Design review of the part built by this model. Coordinates are the model's own, in mm. Round coordinates to 2 decimals unless told otherwise and drop trailing zeros. Write each loop counter-clockwise with the first axis right and the second up, starting at its lowest first coordinate (ties: lowest second). Pieces come first, ordered by that corner, then holes. Notation, with made-up numbers: (55.25, 67.5) -> (61.25, 67.5) arc R23 cw to (61.25, 83.5) -> close; hole circle Ø9 at (-37, 53.5). An arc over 180 degrees is marked (long way). One line per question, with ' | ' between items. Start each with the question number.
1) Consider section A-A (y = -7). Give the boundary of the cut face in (x, z), then the cut area to 3 significant figures.
2) Consider section D-D (y = -53). Give the boundary of the cut face in (x, z).
3) Consider section C-C (x = -2.5). Give the boundary of the cut face in (y, z), then the cut area to 3 significant figures.
4) Mouldability with a two-part tool opening along X and no side actions: class faces 1 (the flat face through (-2, -35, 6)), 2 (the cylindrical face through (-51.225, -1.504, 3.052)), 3 (the flat face through (43.21, -29.65, -40.92)) as +X half, -X half, draft (parallel to the pull), parting line (faces both ways), or undercut.
5) Consider section B-B (z = 1). Give the boundary of the cut face in (x, y).
6) Insertion check: pin 1 Ø25 at (x, z) = (-9, 15.5) entering from -Y; pin 2 Ø4 at (x, y) = (-33.5, -37.5) entering from -Z. Each pin has a flat end and moves straight along its axis. Give the tip position at first contact, or say it passes through.
7) For probe 1 along Y at (x, z) = (-12.5, -2); probe 2 along Z at (x, y) = (17, -49); probe 3 along X at (y, z) = (-54, 8.5), list the stretches that pass through material, from the lowest coordinate up.
```python
from build123d import *

# Parameters (mm, degrees)
F1_DEPTH = 60
F2_R     = 5
F3_R     = 25
F4_DEPTH = 25


with BuildPart() as f1:
    # F0 (on Front) → F1 (new body)
    with BuildSketch(Plane.XZ):
        with BuildLine():
            Line((33.469399, 53.402335), (-27.650935, 53.402335))
            ThreePointArc((-27.650935, 53.402335), (-45.328605, 46.080005), (-52.650935, 28.402335))
            Line((-52.650935, 28.402335), (-52.650935, -21.597665))
            ThreePointArc((-52.650935, -21.597665), (-45.328605, -39.275334), (-27.650935, -46.597665))
            Line((-27.650935, -46.597665), (39.180679, -46.597665))
            Line((39.180679, -46.597665), (47.349065, -35.087663))
            Line((47.349065, -35.087663), (47.349065, 40.44798))
            Line((47.349065, 40.44798), (33.469399, 53.402335))
        make_face()
    extrude(amount=F1_DEPTH)

    # F2
    f2_edges = [f1.edges().sort_by_distance(p)[0] for p in [
        (40.409232, -60, 46.925158),
        (2.909232, -60, 53.402335),
        (-45.328605, -60, 46.080005),
        (-52.650935, -60, 3.402335),
        (-45.328605, -60, -39.275334),
        (5.764872, -60, -46.597665),
        (43.264872, -60, -40.842664),
        (47.349065, -60, 2.680159),
        (40.409232, 0, 46.925158),
        (2.909232, 0, 53.402335),
        (-45.328605, 0, 46.080005),
        (-52.650935, 0, 3.402335),
        (-45.328605, 0, -39.275334),
        (5.764872, 0, -46.597665),
        (43.264872, 0, -40.842664),
        (47.349065, 0, 2.680159),
    ]]
    fillet(f2_edges, radius=F2_R)

    # F3 (on face) → F4 (cut)
    with BuildSketch(Plane.XZ.offset(60)):
        with Locations((-2.058923, 5.945201)):
            Circle(F3_R)
    extrude(amount=-F4_DEPTH, mode=Mode.SUBTRACT)


solid = f1.part
```
From the geometry:
1) outline: (-52.65, -21.6) arc R25 ccw to (-27.65, -46.6) -> (39.18, -46.6) -> (47.35, -35.09) -> (47.35, 40.45) -> (33.47, 53.4) -> (-27.65, 53.4) arc R25 ccw to (-52.65, 28.4) -> close | area: 9,590 mm2
2) outline: (-52.65, -21.6) arc R25 ccw to (-27.65, -46.6) -> (39.18, -46.6) -> (47.35, -35.09) -> (47.35, 40.45) -> (33.47, 53.4) -> (-27.65, 53.4) arc R25 ccw to (-52.65, 28.4) -> close; hole circle Ø50 at (-2.06, 5.95)
3) outline: (-60, -41.6) arc R5 ccw to (-55, -46.6) -> (-5, -46.6) arc R5 ccw to (0, -41.6) -> (0, 48.4) arc R5 ccw to (-5, 53.4) -> (-55, 53.4) arc R5 ccw to (-60, 48.4) -> (-60, 30.94) -> (-35, 30.94) -> (-35, -19.05) -> (-60, -19.05) -> close | area: 4,730 mm2
4) face 1: undercut | face 2: -X half | face 3: +X half
5) outline: (-52.65, -55) arc R5 ccw to (-47.65, -60) -> (-26.56, -60) -> (-26.56, -35) -> (22.45, -35) -> (22.45, -60) -> (42.35, -60) arc R5 ccw to (47.35, -55) -> (47.35, -5) arc R5 ccw to (42.35, 0) -> (-47.65, 0) arc R5 ccw to (-52.65, -5) -> close
6) pin 1: stops at y = -35 | pin 2: stops at z = -46.3
7) probe 1: y = -35 to 0 | probe 2: z = -46.6 to -10.23, 22.12 to 53.4 | probe 3: x = -52.65 to -26.93, 22.81 to 47.35
